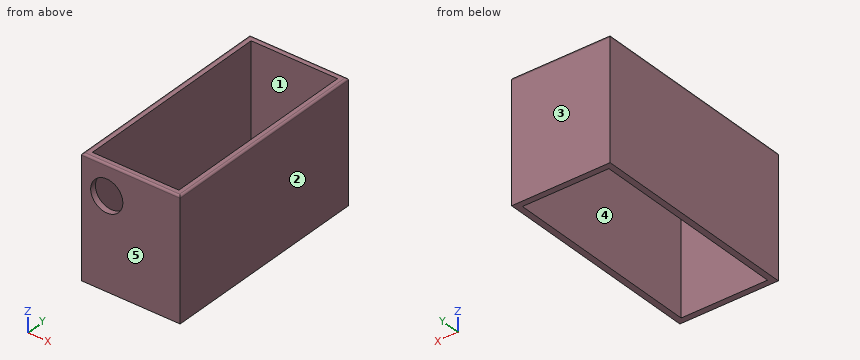
```python
from build123d import *

# Parameters (mm, degrees)
SKETCH_W        = 49
SKETCH_H        = 106
PAD_DEPTH       = 60
SKETCH001_W     = 43
SKETCH001_H     = 100
POCKET_DEPTH    = 60.001
FILLET_R        = 1
SKETCH002_R     = 8
POCKET001_DEPTH = 3


with BuildPart() as part:
    # Sketch → Pad (new body)
    with BuildSketch(Plane.XY):
        Rectangle(SKETCH_W, SKETCH_H)
    extrude(amount=PAD_DEPTH)

    # Sketch001 → Pocket (cut, through all)
    with BuildSketch(Plane.XY.offset(60)):
        Rectangle(SKETCH001_W, SKETCH001_H)
    extrude(amount=-POCKET_DEPTH, mode=Mode.SUBTRACT)

    # Fillet
    fillet_edges = [part.edges().sort_by_distance(p)[0] for p in [
        (0, 53, 60),
        (24.5, 0, 60),
        (-24.5, 0, 60),
        (0, -53, 60),
    ]]
    fillet(fillet_edges, radius=FILLET_R)

    # Sketch002 → Pocket001 (cut)
    with BuildSketch(Plane.XZ.offset(53)):
        with Locations((-12, 45)):
            Circle(SKETCH002_R)
    extrude(amount=-POCKET001_DEPTH, mode=Mode.SUBTRACT)


solid = part.part
```
The model under review builds one solid part; all positions refer to its coordinate system, in mm. Face numbers are marked on the shaded views. A direction names the side the tool comes from. Round coordinates to 2 decimals unless told otherwise and drop trailing zeros. Order: outer loops, then holes, each group sorted by start corner. A loop starts at its lowest first (then second) coordinate and runs counter-clockwise, first axis right, second up. Notation, with made-up numbers: (41, -9.75) -> (100, -9.75) arc R32 cw to (100, 16.25) -> close; hole circle Ø7 at (1, -28.5). An arc over 180 degrees is marked (long way). One line per item, written item: value. Start each with the question number.
Q1. Take a section at C-C (x = -12). Write out the cut boundary in (y, z).
Q2. Take a section at A-A (x = -1). Write out the cut boundary in (y, z).
Q3. Mouldability with a two-part tool opening along X and no side actions: class the marked faces 1, 2 and 3 as released by +X, released by -X, zero draft, split by the parting line, or undercut.
Q4. Machinability: for the marked faces 4 and 5, which of the approach directions +Z, -Z, +X, -X, +Y, -Y give a long, thin tool a straight path to every point of the face, cutting with its end or side? Answer none if there is none.
Q5. Wall thickness on line 1 (Y direction, x = 16, z = 49); line 2 (Z direction, x = -12, y = -51.45); line 3 (X direction, y = -41, z = 6.5): over which ranges is each line inside the solid? List them lowest first.
Q6. Take a section at B-B (y = 34.5). Write out the cut boundary in (x, z).
Q7. Take a section at D-D (z = 45). Write out the cut boundary in (x, y), and give its area (3 significant figures).
Reported:
1. outline: (-53, 0) -> (-50, 0) -> (-50, 37) -> (-53, 37) -> close; (-53, 53) -> (-50, 53) -> (-50, 60) -> (-52, 60) arc R1 ccw to (-53, 59) -> close; (50, 0) -> (53, 0) -> (53, 59) arc R1 ccw to (52, 60) -> (50, 60) -> close
2. outline: (-53, 0) -> (-50, 0) -> (-50, 60) -> (-52, 60) arc R1 ccw to (-53, 59) -> close; (50, 0) -> (53, 0) -> (53, 59) arc R1 ccw to (52, 60) -> (50, 60) -> close
3. face 1: undercut
3. face 2: released by +X
3. face 3: zero draft
4. face 4: +Z, -Z
4. face 5: +Z, -Z, +X, -X, -Y
5. line 1: y = -53 to -50, 50 to 53
5. line 2: z = 0 to 37, 53 to 60
5. line 3: x = -24.5 to -21.5, 21.5 to 24.5
6. outline: (-24.5, 0) -> (-21.5, 0) -> (-21.5, 60) -> (-23.5, 60) arc R1 ccw to (-24.5, 59) -> close; (21.5, 0) -> (24.5, 0) -> (24.5, 59) arc R1 ccw to (23.5, 60) -> (21.5, 60) -> close
7. outline: (-24.5, -53) -> (-20, -53) -> (-20, -50) -> (-21.5, -50) -> (-21.5, 50) -> (21.5, 50) -> (21.5, -50) -> (-4, -50) -> (-4, -53) -> (24.5, -53) -> (24.5, 53) -> (-24.5, 53) -> close
7. area: 846 mm2
